Geometry: see drawing. Coordinates: mm, zero at the bounding-box minimum. A direction names the side the tool comes from. Give positions to 0.01 mm unless a question says otherwise; leave off trailing zeros. Order: outer loops, then holes, each group sorted by start corner. A loop starts at its lowest first (then second) coordinate and runs counter-clockwise, first axis right, second up. Notation, with made-up numbers: M -35,-1.5 L 23,-1.5 A8 cw 23,12.5 Z; hole C 75,40 d8. An arc over 180 degrees is marked long. Use a Markdown table: item, result.
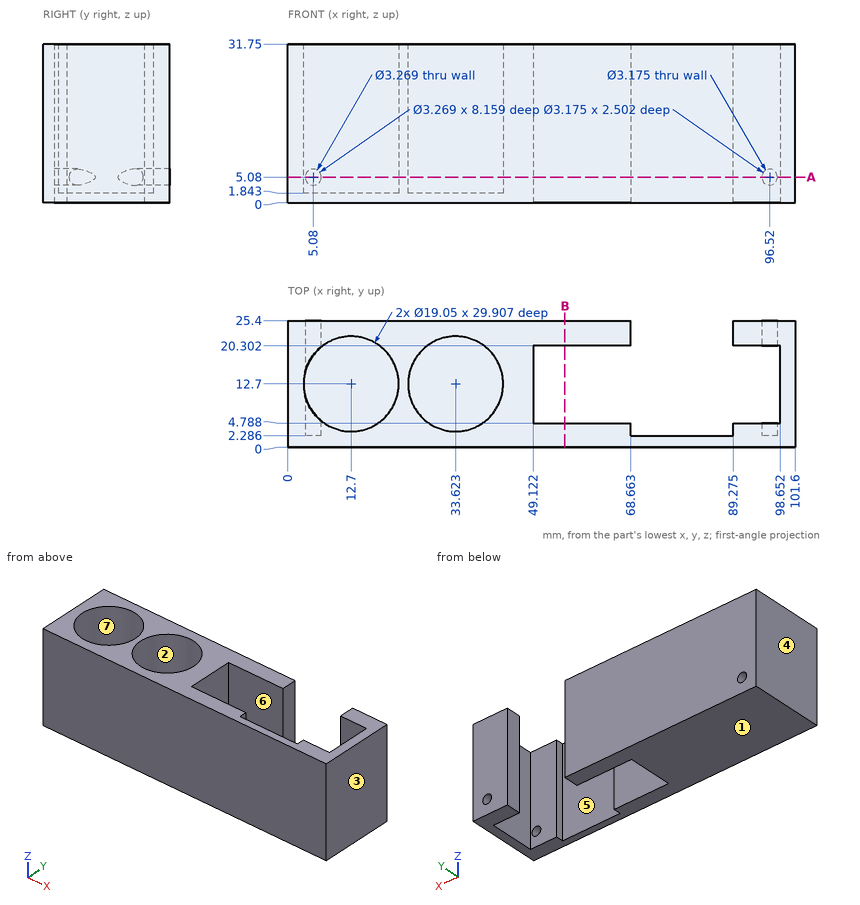
1) Mould query, pull axis X, two halves, no side actions, for the marked faces 1, 2, 3 and 4. Classes: released by +X, released by -X, zero draft, split by the parting line, or undercut.
Response values:
| item | result |
|---|---|
| face 1 | zero draft |
| face 2 | undercut |
| face 3 | released by +X |
| face 4 | released by -X |
2) Cut plane A-A on z = 5.08. State how many separate pieces and enclosed holes the cut face has, and give its area (3 significant figures).
Response values:
| item | result |
|---|---|
| separate pieces | 2 |
| enclosed holes | 1 |
| area | 1,020 mm² |
3) Cut plane B-B on x = 55.5. Return loops of the section in (y, z), and give its area (3 significant figures).
Response values:
| item | result |
|---|---|
| outline | M 0,0 L 4.79,0 L 4.79,31.75 L 0,31.75 Z; M 20.3,0 L 25.4,0 L 25.4,31.75 L 20.3,31.75 Z |
| area | 314 mm² |
4) First-contact query: pin 1 Ø1 at (x, z) = (5, 6) entering from +Y; pin 2 Ø5.5 at (x, y) = (16, 14.5) entering from +Z. Flat tips, straight axial feed; report the tip coordinate or a pass-through.
Response values:
| item | result |
|---|---|
| pin 1 | stops at y = 2.29 |
| pin 2 | stops at z = 1.84 |
5) Reachability of the marked faces 5, 6 and 7 from +Z, -Z, +X, -X, +Y, -Y: full face, straight path, thin tool, end or side. Return the list, or none.
Response values:
| item | result |
|---|---|
| face 5 | +Z, -Z, +Y |
| face 6 | +Z, -Z |
| face 7 | +Z |
6) Material intervals for line 1 (Y direction, x = 54, z = 23); line 2 (Z direction, x = 96.52, y = 22.3); line 3 (X direction, y = 18.5, z = 8) (1 decimal), sorted ascending. Write a range as from..to.
Response values:
| item | result |
|---|---|
| line 1 | y = 0..4.79, 20.3..25.4 |
| line 2 | z = 0..3.49, 6.67..31.75 |
| line 3 | x = 0..5.1, 20.3..26.1, 41.2..49.1, 98.7..101.6 |
